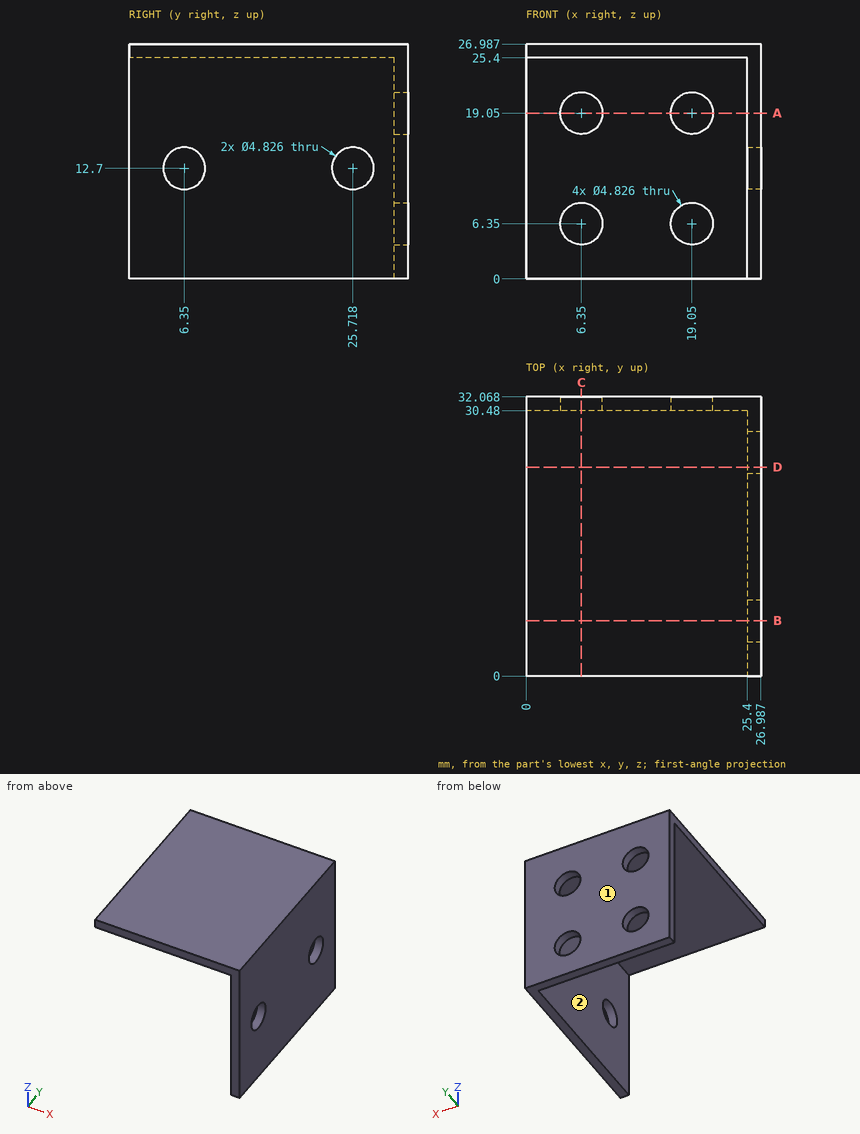
Part print with two shaded views. Sizes in mm from the minimum x, y, z corner. A direction names the side the tool comes from. Round coordinates to 2 decimals unless told otherwise and drop trailing zeros. Order: outer loops, then holes, each group sorted by start corner. A loop starts at its lowest first (then second) coordinate and runs counter-clockwise, first axis right, second up. Notation, with made-up numbers: (5, -23.75) -> (61, -23.75) arc R6 ccw to (61, -13.75) -> close; hole circle Ø9 at (-13.5, 0). An arc over 180 degrees is marked (long way). Write each question's results on one line, items separated by ' | '.
1. Cut at D-D (y = 24). Give the cut face in (x, z) (1 decimal).
Findings below:
outline: (0, 25.4) -> (25.4, 25.4) -> (25.4, 14.4) -> (27, 14.4) -> (27, 27) -> (0, 27) -> close; (25.4, 0) -> (27, 0) -> (27, 11) -> (25.4, 11) -> close
2. Cut at A-A (z = 19.05). Give the cut face in (x, y).
Findings below:
outline: (0, 30.48) -> (3.94, 30.48) -> (3.94, 32.07) -> (0, 32.07) -> close; (8.76, 30.48) -> (16.64, 30.48) -> (16.64, 32.07) -> (8.76, 32.07) -> close; (21.46, 30.48) -> (25.4, 30.48) -> (25.4, 0) -> (26.99, 0) -> (26.99, 32.07) -> (21.46, 32.07) -> close
3. 3-axis set-ups, long thin cutter, end or side, ignore diameter. For the marked faces 1 and 2: which of +Z, -Z, +X, -X, +Y, -Y reach the whole face in a straight line?
Findings below:
face 1: +Z, -Z, +X, -X, +Y | face 2: -Z, -X, -Y
4. Flat gauge pins, fed straight in: P1, Ø7.5, axis at x = 6.35, z = 19.05, coming from the -Y side; P2, Ø6.5, axis at y = 6.35, z = 12.7, coming from the -X side; P3, Ø4.5, axis at x = 6.35, z = 6.35, coming from the -Y side; P4, Ø6, axis at x = 17, y = 22, coming from the -Z side. Where does each tip first touch, or does it go through?
Findings below:
P1: stops at y = 30.48 | P2: stops at x = 25.4 | P3: passes through | P4: stops at z = 25.4
5. Cut at B-B (y = 6.35). Give the cut face in (x, z).
Findings below:
outline: (0, 25.4) -> (25.4, 25.4) -> (25.4, 15.11) -> (26.99, 15.11) -> (26.99, 26.99) -> (0, 26.99) -> close; (25.4, 0) -> (26.99, 0) -> (26.99, 10.29) -> (25.4, 10.29) -> close
6. Wall check: line 1 along Y through (x, z) = (26.4, 12.7) (1 decimal); line 2 along Z through (x, y) = (19.05, 31.45); line 3 along Y through (x, z) = (5, 25). Give the ranges that are in metal, low to high. Write a range as [from, to].
Findings below:
line 1: y = [0, 3.9], [8.8, 23.3], [28.1, 32.1] | line 2: z = [0, 3.94], [8.76, 16.64], [21.46, 26.99] | line 3: y = [30.48, 32.07]
7. Cut at C-C (x = 6.35). Give the cut face in (y, z).
Findings below:
outline: (0, 25.4) -> (30.48, 25.4) -> (30.48, 21.46) -> (32.07, 21.46) -> (32.07, 26.99) -> (0, 26.99) -> close; (30.48, 0) -> (32.07, 0) -> (32.07, 3.94) -> (30.48, 3.94) -> close; (30.48, 8.76) -> (32.07, 8.76) -> (32.07, 16.64) -> (30.48, 16.64) -> close
